from build123d import *

# Parameters (mm, degrees)
F0_W     = 69.85
F0_H     = 44.45
F1_DEPTH = 25.4
F3_DEPTH = 12.7
F4_R     = 14.840288
F5_DEPTH = 25.401


with BuildPart() as f1:
    # F0 (on Front) → F1 (new body)
    with BuildSketch(Plane.XZ):
        with Locations((34.925, 22.225)):
            Rectangle(F0_W, F0_H)
    extrude(amount=F1_DEPTH)

    # F2 (on Front) → F3 (cut, symmetric)
    with BuildSketch(Plane.XZ):
        Polygon((69.931224, 45.74215), (19.692384, 44.191573), (54.735523, 0), (69.931224, 0), align=None)
    extrude(amount=F3_DEPTH, both=True, mode=Mode.SUBTRACT)

    # F4 (on Front) → F5 (cut, through all)
    with BuildSketch(Plane.XZ):
        with Locations((19.692384, 24.344128)):
            Circle(F4_R)
    extrude(amount=F5_DEPTH, mode=Mode.SUBTRACT)


solid = f1.part
Verification items for the finished model (mm, model axes). A direction names the side the tool comes from. Coordinates: 2 decimals unless noted, no trailing zeros. Write each loop counter-clockwise with the first axis right and the second up, starting at its lowest first coordinate (ties: lowest second). Pieces come first, ordered by that corner, then holes. Notation, with made-up numbers: M -17.5,10.25 L 32.5,10.25 A24 cw 32.5,44.25 Z; hole C 6,-35.5 d4. An arc over 180 degrees is marked long. One line per question, with ' | ' between items.
1) Sectioned sample at A-A on y = -9. Record the cut outline in (x, z), then the cut area to 3 significant figures.
Solutions:
outline: M 0,0 L 54.74,0 L 34.48,25.54 A14.84 cw long 24.23,38.48 L 19.69,44.19 L 28.07,44.45 L 0,44.45 Z | area: 987 mm^2
2) Sectioned sample at D-D on y = -15.25. Record the cut outline in (x, z), then the cut area to 3 significant figures.
Solutions:
outline: M 0,0 L 69.85,0 L 69.85,44.45 L 0,44.45 Z; hole C 19.69,24.34 d29.68 | area: 2,410 mm^2
3) Access from +Z, -Z, +X, -X, +Y, -Y to the whole of each face (thin tool, end or side, straight path). Record for faces 1 (the face through (44.468, -6.439, 12.948)), 2 (the face through (0, -13, 22)).
Solutions:
face 1: +Z, +X, +Y | face 2: +Z, -Z, -X, +Y, -Y
4) Release check for a two-part mould opening along Z. For faces 3 (the face through (27, -15, 44.45)), 4 (the face through (69.85, -19, 22)), 5 (the face through (21.93, -6.44, 41.37)) record: +Z half, -Z half, draft (parallel to the pull), parting line (faces both ways), or undercut.
Solutions:
face 3: +Z half | face 4: draft | face 5: undercut
5) Depth check by flat-ended pin: pin 1 Ø5 at (x, y) = (18.5, -16.5) entering from -Z; pin 2 Ø12 at (x, y) = (60, -5) entering from +Z; pin 3 Ø22 at (x, z) = (54, 23) entering from +Y. Enter the tip coordinate at first touch or a pass-through.
Solutions:
pin 1: z = 0 | pin 2: z = 0.93 | pin 3: y = -12.7
6) Sectioned sample at B-B on z = 19.5. Record the cut outline in (x, y), then the cut area to 3 significant figures.
Solutions:
outline: M 0,-25.4 L 5.66,-25.4 L 5.66,0 L 0,0 Z; M 33.72,-25.4 L 69.85,-25.4 L 69.85,-12.7 L 39.27,-12.7 L 39.27,0 L 33.72,0 Z | area: 673 mm^2
7) Material ranges on L1, parallel to X at y = -22.25, z = 24.5; L2, parallel to Y at x = 35, z = 29; L3, parallel to X at y = -13.75, z = 18, recorded low to high.
Solutions:
L1: 0 to 4.85, 34.53 to 69.85 | L2: -25.4 to -12.7 | L3: 0 to 6.28, 33.11 to 69.85
8) Sectioned sample at C-C on x = 32. Record the cut outline in (y, z), then the cut area to 3 significant figures.
Solutions:
outline: M -25.4,0 L 0,0 L 0,16.05 L -25.4,16.05 Z; M -25.4,32.64 L -12.7,32.64 L -12.7,44.45 L -25.4,44.45 Z | area: 558 mm^2
